Here's how the part is built. I have some questions about the finished solid (model axes, mm). Round coordinates to 2 decimals unless told otherwise and drop trailing zeros. Loops run counter-clockwise (first coordinate to the right, second up) from the corner with the lowest first, then second, coordinate; pieces in that order, holes last. Notation, with made-up numbers: M 58,56.25 L 64,56.25 A36 ccw 64,90.25 Z; hole C 56,-11 d8. An arc over 180 degrees is marked long. Write item = value, one per line. Start each with the question number.
Autodesk Inventor part; units mm, degrees
ref_plane "YZ Plane" through (0, 0, 0) normal (1, 0, 0) x (0, 1, 0)
ref_plane "XZ Plane" through (0, 0, 0) normal (0, 1, 0) x (-1, 0, 0)
ref_plane "XY Plane" through (0, 0, 0) normal (0, 0, 1) x (1, 0, 0)
sketch "Sketch2" plane through (0, 0, 0) normal (0, 1, 0) x (-1, 0, 0)
  line L0 (-27.5, -23.5) -> (27.5, -23.5)
  line L1 (27.5, -23.5) -> (27.5, 23.5)
  line L2 (27.5, 23.5) -> (-27.5, 23.5)
  line L3 (-27.5, 23.5) -> (-27.5, -23.5)
  line L4 (-27.5, -23.5) -> (27.5, 23.5) construction
  line L5 (27.5, -23.5) -> (-27.5, 23.5) construction
  line L6 (27.5, -10.8102) -> (-21.5, 23.5)
  line L7 (-12.5, -23.5) -> (-27.5, 11.5)
  point P0 (0, 0)
  dimension "d1" = 55
  dimension "d2" = 47
  dimension "d3" = 15
  dimension "d4" = 6
  dimension "d5" = 35
  dimension "d28" = 35
  dimension "d29" = 12.6898
extrude "Extrusion1" add sketch "Sketch2" along normal mid plane 16 contours L7 L3 L2 L6 L1 L0
sketch "Sketch3" plane through (0, -8, 0) normal (0, -1, 0) x (1, 0, 0)
  line L0 (-27.5, -23.5) -> (12.5, -23.5)
  line L1 (27.5, 11.5) -> (27.5, 23.5)
  point P0 (0, 0)
  point P1 (12.5, 1.5)
  dimension "d9" = 25
  dimension "d10" = 15
hole "Hole1" at (12.5, -8, 1.5) direction (0, 1, 0) diameter 10 end through all
sketch "Sketch4" plane through (0, -8, 0) normal (0, -1, 0) x (1, 0, 0)
  line L0 (-27.5, -23.5) -> (12.5, -23.5)
  line L1 (27.5, 11.5) -> (27.5, 23.5)
  point P0 (0, 0)
  point P1 (-17.5, -13.5)
  dimension "d18" = 10
  dimension "d19" = 45
hole "Hole2" at (-17.5, -8, -13.5) direction (0, 1, 0) diameter 6.647 end through all
fillet "Fillet1" radius 5 1 edges at (12.5, 0, -23.5)
properties part number "TL20240701-10100AT-003" material "MC NYLON"
Item 1: We'd pull the mould along X, two halves only. Please class faces 1 (the cylindrical face through (-20.8, 0.1, -13.1)), 2 (the flat face through (20.553, -0.112, -4.709)), 3 (the flat face through (0, 8, -5)): released by +X, released by -X, zero draft, split by the parting line, or undercut.
Item 2: Please list where these lines run through material, in increasing order: line 1 (X direction, y = -3, z = 1.5); line 2 (Z direction, x = 12.5, y = 4); line 3 (Z direction, x = 8, y = 5.75). Write a range as [from, to].
Item 3: Will these pins go through, and if not, where does the flat tip stop? pin 1 Ø8 at (x, z) = (12.5, 1.5) entering from -Y; pin 2 Ø8 at (y, z) = (1, -15) entering from +X; pin 3 Ø8 at (y, z) = (-5.5, -10.5) entering from +X; pin 4 Ø8 at (y, z) = (3.5, 6.5) entering from +X.
Item 4: I want a section at D-D, the plane z = -8. List the corners of the cut face in (x, y) for me.
Item 5: I want a section at A-A, the plane x = 12.5. List the corners of the cut face in (y, z) for me.
Item 6: I want a section at C-C, the plane y = -1.75. List the corners of the cut face in (x, z) for me.
Item 7: I want a section at B-B, the plane z = -13.5. List the corners of the cut face in (x, y) for me, then the cut area to 3 significant figures.
Worked out:
q1.face_1 = undercut
q1.face_2 = released by +X
q1.face_3 = zero draft
q2.line_1 = [-9.92, 7.5], [17.5, 23.21]
q2.line_2 = [-22.26, -3.5], [6.5, 17.2]
q2.line_3 = [-23.5, -0.68], [3.68, 14.05]
q3.pin_1 = through
q3.pin_2 = 17.86
q3.pin_3 = 19.79
q3.pin_4 = 27.07
q4.outline = M -23.49,-8 L 19.14,-8 L 19.14,8 L -23.49,8 Z
q5.outline = M -8,-22.26 L 8,-22.26 L 8,-3.5 L -8,-3.5 Z; M -8,6.5 L 8,6.5 L 8,17.2 L -8,17.2 Z
q6.outline = M -27.5,-23.5 L 9.2,-23.5 A5 ccw 13.8,-20.47 L 27.5,11.5 L 27.5,23.5 L 21.5,23.5 L -27.5,-10.81 Z; hole C -17.5,-13.5 d6.65; hole C 12.5,1.5 d10
q7.outline = M -27.5,-8 L -20.82,-8 L -20.82,8 L -27.5,8 Z; M -14.18,-8 L 16.79,-8 L 16.79,8 L -14.18,8 Z
q7.area = 602 mm2
